from build123d import *

# Parameters (mm, degrees)
F0_R     = 1.8288
F1_DEPTH = 6.35
F2_R     = 2.54


with BuildPart() as f1:
    # F0 (on Front) → F1 (new body)
    with BuildSketch(Plane.XZ):
        with BuildLine():
            Line((-4.318172, -17.96034), (-1.524, -17.96034))
            Line((-1.524, -17.96034), (-1.524, -7.94766))
            ThreePointArc((-1.524, -7.94766), (0, -6.42366), (1.524, -7.94766))
            Line((1.524, -7.94766), (1.524, -17.96034))
            Line((1.524, -17.96034), (4.318172, -17.96034))
            ThreePointArc((4.318172, -17.96034), (8.313921, -8.313921), (17.96034, -4.318172))
            Line((17.96034, -4.318172), (17.96034, -1.524))
            Line((17.96034, -1.524), (7.94766, -1.524))
            ThreePointArc((7.94766, -1.524), (6.42366, 0), (7.94766, 1.524))
            Line((7.94766, 1.524), (17.96034, 1.524))
            Line((17.96034, 1.524), (17.96034, 4.318172))
            ThreePointArc((17.96034, 4.318172), (8.313921, 8.313921), (4.318172, 17.96034))
            Line((4.318172, 17.96034), (1.524, 17.96034))
            Line((1.524, 17.96034), (1.524, 7.94766))
            ThreePointArc((1.524, 7.94766), (0, 6.42366), (-1.524, 7.94766))
            Line((-1.524, 7.94766), (-1.524, 17.96034))
            Line((-1.524, 17.96034), (-4.318172, 17.96034))
            ThreePointArc((-4.318172, 17.96034), (-8.313921, 8.313921), (-17.96034, 4.318172))
            Line((-17.96034, 4.318172), (-17.96034, 1.524))
            Line((-17.96034, 1.524), (-7.94766, 1.524))
            ThreePointArc((-7.94766, 1.524), (-6.42366, 0), (-7.94766, -1.524))
            Line((-7.94766, -1.524), (-17.96034, -1.524))
            Line((-17.96034, -1.524), (-17.96034, -4.318172))
            ThreePointArc((-17.96034, -4.318172), (-8.313921, -8.313921), (-4.318172, -17.96034))
        make_face()
        with Locations((4.490128, -4.490128)):
            Circle(F0_R, mode=Mode.SUBTRACT)
        with Locations((-4.490128, 4.490128)):
            Circle(F0_R, mode=Mode.SUBTRACT)
    extrude(amount=F1_DEPTH)

    # F2
    f2_edges = [f1.edges().sort_by_distance(p)[0] for p in [
        (-1.524, -3.175, -17.96034),
        (1.524, -3.175, -17.96034),
        (-17.96034, -3.175, 1.524),
        (17.96034, -3.175, 1.524),
        (-17.96034, -3.175, -1.524),
        (17.96034, -3.175, -1.524),
        (1.524, -3.175, 17.96034),
        (-1.524, -3.175, 17.96034),
    ]]
    fillet(f2_edges, radius=F2_R)


solid = f1.part
Can you work these out from the model? Positions are in its coordinate system, mm. A direction names the side the tool comes from. Coordinates: 2 decimals unless noted, no trailing zeros. Write each loop counter-clockwise with the first axis right and the second up, starting at its lowest first coordinate (ties: lowest second). Pieces come first, ordered by that corner, then holes. Notation, with made-up numbers: (14, 86) -> (44, 86) arc R24 ccw to (44, 105) -> close; hole circle Ø2 at (86, -32.5). An arc over 180 degrees is marked (long way). Write each question's results on one line, items separated by ' | '. Start each with the question number.
Item 1: Please list where these lines run through material, in increasing order: probe 1 along Z at (x, y) = (16.5, -2); probe 2 along Z at (x, y) = (-9.5, -1.25); probe 3 along X at (y, z) = (-4, -15).
Item 2: On a 3-axis mill with a long thin cutter (end or side, diameter ignored), from which of +Z, -Z, +X, -X, +Y, -Y can I reach the whole of each face in a straight line? I mean faces 1 (the flat face through (-12, -3, 1.524)), 2 (the cylindrical face through (17.24, -3.22, -2.29)), 3 (the cylindrical face through (-2.29, -3.22, -17.24)), 4 (the cylindrical face through (-2.29, -3.22, 17.24)). Say none if no direction works.
Item 3: I'm going to push flat-ended pins straight in: P1, Ø3, axis at x = -8, y = -3, coming from the +Z side; P2, Ø3, axis at x = 12, y = -2.5, coming from the +Z side; P3, Ø1.9, axis at y = -4.5, z = 10, coming from the +X side; P4, Ø3, axis at x = 3, z = 5.5, coming from the +Y side. Where does each tip first touch, or does it pass through?
Item 4: If we section it at A-A, the plane z = -8.5: Write out the boundary of the cut face in (x, y).
Item 5: If we section it at C-C, the plane y = -4.5: Count the separate pieces of the cut face and the enclosed holes in it, and give its area (3 significant figures).
Item 6: If we section it at D-D, the plane x = 0: Write out the boundary of the cut face in (y, z).
Item 7: If we section it at B-B, the plane x = 5: Write out the boundary of the cut face in (y, z).
Item 8: Thinking about a two-plate mould opening in Z: for faces 5 (the cylindrical face through (-3.507, -3.131, 6.032)), 6 (the cylindrical face through (2.25, -3.22, 17.2)), 7 (the cylindrical face through (-17.2, -3.22, 2.25)), 8 (the flat face through (1.524, -3, -12)), which applies, released by +Z, released by -Z, zero draft, split by the parting line, or undercut?
Answer block:
1) probe 1: -4.4 to -1.76, 1.76 to 4.4 | probe 2: -7.26 to -1.52, 1.52 to 7.26 | probe 3: -4.64 to -1.52, 1.52 to 4.64
2) face 1: -X, +Y, -Y | face 2: +X, +Y, -Y | face 3: -Z, +Y, -Y | face 4: +Z, +Y, -Y
3) P1: z = 10.56 | P2: z = 6.54 | P3: x = 7.63 | P4: y = 0
4) outline: (-8.13, -6.35) -> (-1.52, -6.35) -> (-1.52, 0) -> (-8.13, 0) -> close; (1.52, -6.35) -> (8.13, -6.35) -> (8.13, 0) -> (1.52, 0) -> close
5) separate pieces: 1 | enclosed holes: 2 | area: 537 mm²
6) outline: (-6.35, -6.42) -> (0, -6.42) -> (0, 6.42) -> (-6.35, 6.42) -> close
7) outline: (-6.35, -13.7) -> (0, -13.7) -> (0, -6.25) -> (-6.35, -6.25) -> close; (-6.35, -2.73) -> (0, -2.73) -> (0, 13.7) -> (-6.35, 13.7) -> close
8) face 5: undercut | face 6: released by +Z | face 7: undercut | face 8: zero draft
